The listing builds one solid part. Answer for the finished solid, in the listing's coordinates (mm). A direction names the side the tool comes from. Coordinates: 2 decimals unless noted, no trailing zeros. Write each loop counter-clockwise with the first axis right and the second up, starting at its lowest first coordinate (ties: lowest second). Pieces come first, ordered by that corner, then holes. Notation, with made-up numbers: M 52.5,-9.75 L 106.5,-9.75 A25 cw 106.5,11.25 Z; hole C -2,16.5 d6. An arc over 180 degrees is marked long. Put each result on its own line as item: value. Start each with the question number.
```python
from build123d import *

# Parameters (mm, degrees)
BOSS_EXTRUDE2_DEPTH = 5
SKETCH23_W          = 2
SKETCH23_H          = 1
CUT_EXTRUDE16_DEPTH = 5
CUT_EXTRUDE17_DEPTH = 7
SKETCH25_W          = 2
SKETCH25_H          = 2
SKETCH25_H_2        = 3
BOSS_EXTRUDE5_DEPTH = 5
CUT_EXTRUDE18_DEPTH = 2
CUT_EXTRUDE19_DEPTH = 2


with BuildPart() as part:
    # Sketch7 → Boss-Extrude2 (new body)
    with BuildSketch(Plane.XY):
        Polygon((0, 0), (0, 5), (6, 5), (6, 0), (4, 0), (4, 1), (2, 1), (2, 0), align=None)
    extrude(amount=BOSS_EXTRUDE2_DEPTH)

    # Sketch23 → Cut-Extrude16 (cut)
    with BuildSketch(Plane(origin=(0, 5, 0), x_dir=(1, 0, 0), z_dir=(0, 1, 0))):
        with Locations((3, -4.5)):
            Rectangle(SKETCH23_W, SKETCH23_H)
    extrude(amount=-CUT_EXTRUDE16_DEPTH, mode=Mode.SUBTRACT)

    # Sketch24 → Cut-Extrude17 (cut)
    with BuildSketch(Plane.ZY):
        Polygon((0, 5), (4, 1), (4, 5), align=None)
    extrude(amount=-CUT_EXTRUDE17_DEPTH, mode=Mode.SUBTRACT)

    # Sketch25 → Boss-Extrude5 (add)
    with BuildSketch(Plane.XZ):
        with Locations((1, 4)):
            Rectangle(SKETCH25_W, SKETCH25_H)
        with Locations((5, 3.5)):
            Rectangle(SKETCH25_W, SKETCH25_H_2)
    extrude(amount=-BOSS_EXTRUDE5_DEPTH)

    # Sketch26 → Cut-Extrude18 (cut)
    with BuildSketch(Plane.ZY):
        Polygon((5, 5), (5, 4), (3, 2), (3, 5), align=None)
    extrude(amount=-CUT_EXTRUDE18_DEPTH, mode=Mode.SUBTRACT)

    # Sketch27 → Cut-Extrude19 (cut)
    with BuildSketch(Plane(origin=(6, 0, 0), x_dir=(0, 0, -1), z_dir=(1, 0, 0))):
        Polygon((-5, 5), (-2, 3), (-2, 5), align=None)
    extrude(amount=-CUT_EXTRUDE19_DEPTH, mode=Mode.SUBTRACT)


solid = part.part
```
1) For faces 4 (the face through (1, 3, 4)), 5 (the face through (4, 2, 4)), 6 (the face through (5, 4, 3.5)), 7 (the face through (3, 1, 2)), determine the directions among +Z, -Z, +X, -X, +Y, -Y from which every point of the face is accessible in a straight line to the end or side of a thin tool.
2) A cutting plane is placed at A-A on y = 2.5. Write down the section's boundary in (x, z).
3) A cutting plane is placed at D-D on x = 1.25. Write down the section's boundary in (y, z).
4) A cutting plane is placed at C-C on z = 1.7. Write down the section's boundary in (x, y).
5) Straight lines are drawn through the part: probe 1 along X at (y, z) = (3.35, 4.65); probe 2 along X at (y, z) = (3.65, 3.55); probe 3 along Z at (x, y) = (5, 4.75) (3 decimals). For each, find the intervals that lie inside material, in ascending order.
6) Determine the mould class of faces 1 (the face through (2, 2, 4)), 2 (the face through (6, 2, 2)), 3 (the face through (3, 3, 0)) for opening direction X: +X half, -X half, draft (parallel to the pull), parting line (faces both ways), or undercut.
7) A cutting plane is placed at B-B on z = 4.1. Write down the section's boundary in (x, y), then the cut area to 3 significant figures.
8) Given pin 1 Ø1 at (x, z) = (3, 1) entering from -Y; pin 2 Ø1.5 at (y, z) = (4, 3) entering from -X, each flat-ended and moving along its own axis, determine where each tip first touches the part or whether it passes through.
Answers follow:
1. face 4: -X, +Y
1. face 5: +Z
1. face 6: +X, -X, +Y
1. face 7: +Z, -Z, -Y
2. outline: M 0,0 L 6,0 L 6,5 L 4,5 L 4,2.5 L 0,2.5 Z; M 0,3.5 L 2,3.5 L 2,5 L 0,5 Z
3. outline: M 0,0 L 5,0 L 2,3 L 4,5 L 0,5 Z
4. outline: M 0,0 L 2,0 L 2,1 L 4,1 L 4,0 L 6,0 L 6,3.3 L 0,3.3 Z
5. probe 1: x = 0 to 2, 4 to 6
5. probe 2: x = 4 to 6
5. probe 3: z = 0 to 0.25, 4.625 to 5
6. face 1: undercut
6. face 2: +X half
6. face 3: draft
7. outline: M 0,0 L 2,0 L 2,3.1 L 0,3.1 Z; M 4,0 L 6,0 L 6,4.4 L 4,4.4 Z
7. area: 15.0 mm²
8. pin 1: stops at y = 1
8. pin 2: stops at x = 4
